from build123d import *

# Parameters (mm, degrees)
SALIENTE_EXTRUIR1_DEPTH = 4


with BuildPart() as part:
    # Croquis1 → Saliente-Extruir1 (new, symmetric)
    with BuildSketch(Plane(origin=(0, 54.707138557, 0), x_dir=(1, 0, 0), z_dir=(0, 1, 0))):
        with BuildLine():
            Line((-153.357036721, -77.1), (49.152963279, -77.1))
            Line((49.152963279, -77.1), (49.152963279, -46.00446543))
            Line((49.152963279, -46.00446543), (142.897963279, -46.00446543))
            ThreePointArc((142.897963279, -46.00446543), (159.865368491, -53.032594788), (166.893497848, -70))
            Line((166.893497848, -70), (166.893497848, -460))
            ThreePointArc((166.893497848, -460), (159.865368491, -476.967405212), (142.897963279, -483.99553457))
            Line((142.897963279, -483.99553457), (49.152963279, -483.99553457))
            Line((49.152963279, -483.99553457), (49.152963279, -452.9))
            Line((49.152963279, -452.9), (-153.357036721, -452.9))
            Line((-153.357036721, -452.9), (-153.357036721, -483.99553457))
            Line((-153.357036721, -483.99553457), (-247.102036721, -483.99553457))
            ThreePointArc((-247.102036721, -483.99553457), (-264.069441934, -476.967405212), (-271.097571291, -460))
            Line((-271.097571291, -460), (-271.097571291, -70))
            ThreePointArc((-271.097571291, -70), (-264.069441934, -53.032594788), (-247.102036721, -46.00446543))
            Line((-247.102036721, -46.00446543), (-153.357036721, -46.00446543))
            Line((-153.357036721, -46.00446543), (-153.357036721, -77.1))
        make_face()
    extrude(amount=SALIENTE_EXTRUIR1_DEPTH, both=True)


solid = part.part
Build history of the part. All positions in model axes, mm. Round coordinates to 2 decimals unless told otherwise and drop trailing zeros. Write each loop counter-clockwise with the first axis right and the second up, starting at its lowest first coordinate (ties: lowest second). Pieces come first, ordered by that corner, then holes. Notation, with made-up numbers: M 2.25,18.25 L 49.25,18.25 A20 cw 49.25,22.25 Z; hole C 77,-28.5 d9. An arc over 180 degrees is marked long. Answer as a JSON object with one key per item and string values. Group by question number.
(1) Cut at A-A (y = 53.25). Give the cut face in (x, z).
(2) Drill centre lines: L1, parallel to X at y = 51.5, z = 68.5; L2, parallel to Z at x = 15, y = 55.5; L3, parallel to Z at x = 146, y = 56.5. Where is each one in solid material? Low to high.
(3) Cut at B-B (x = -68.5). Give the cut face in (y, z), and give its area (3 significant figures).
(4) Flat gauge pins, fed straight in: pin 1 (2 mm diameter, centred on x = 43.5, y = 57, fed in from -Z); pin 2 (2.5 mm diameter, centred on y = 53, z = 466, fed in from -X); pin 3 (3 mm diameter, centred on x = -80, y = 56.5, fed in from +Z). Where does each tip first touch, or does it go through?
Responses:
{
 "1": {"outline": "M -271.1,70 A24 ccw -247.1,46 L -153.36,46 L -153.36,77.1 L 49.15,77.1 L 49.15,46 L 142.9,46 A24 ccw 166.89,70 L 166.89,460 A24 ccw 142.9,484 L 49.15,484 L 49.15,452.9 L -153.36,452.9 L -153.36,484 L -247.1,484 A24 ccw -271.1,460 Z"},
 "2": {"L1": "x = -271.05 to -153.36, 49.15 to 166.85", "L2": "z = 77.1 to 452.9", "L3": "z = 46.21 to 483.79"},
 "3": {"outline": "M 50.71,77.1 L 58.71,77.1 L 58.71,452.9 L 50.71,452.9 Z", "area": "3,010 mm2"},
 "4": {"pin 1": "stops at z = 77.1", "pin 2": "stops at x = -270.62", "pin 3": "stops at z = 452.9"}
}
